CAD build for the part. Positions are in the model's coordinates, mm. A direction names the side the tool comes from. Coordinates: 2 decimals unless noted, no trailing zeros. Loops run counter-clockwise (first coordinate to the right, second up) from the corner with the lowest first, then second, coordinate; pieces in that order, holes last. Notation, with made-up numbers: (-38, 52) -> (-8, 52) arc R15 ccw to (-8, 65) -> close; hole circle Ø5 at (-38, 56.25). An arc over 180 degrees is marked (long way). Write item = value, one per line. Start each with the question number.
(1) Band-saw the part on C-C (y = 0). Write the cut outline in (x, z), and give its area (3 significant figures).
(2) Tool access for faces 5 (the face through (0, 21.5, 27)), 6 (the face through (5.109, 22.514, 37.026)): list every direction of +Z, -Z, +X, -X, +Y, -Y with a clear straight run to the whole face (end or side of a thin tool).
(3) Pull direction Z, two halves, no side cores. Call faces 1 (the face through (0, -21.5, 27)), 2 (the face through (-14.246, 22.514, 45.613)), 3 (the face through (0, 0, 0)), 4 (the face through (-10, 23, 49)): +Z half, -Z half, draft (parallel to the pull), parting line (faces both ways), or undercut.
(4) Band-saw the part on D-D (x = 14.25). Write the cut outline in (y, z).
(5) Drill centre lines: line 1 (Y direction, x = 3.5, z = 27); line 2 (Z direction, x = -13, y = 22); line 3 (Y direction, x = 14.25, z = 0.95). Where is each one in solid material? Low to high. Write a range as from..to.
(6) Band-saw the part on A-A (z = 18). Write the cut outline in (x, y).
(7) Flat gauge pins, fed straight in: P1, Ø7, axis at x = -13, z = 40, coming from the +Y side; P2, Ø2, axis at x = -16, y = 8, coming from the +Z side. Where does each tip first touch, or does it go through?
(8) Band-saw the part on B-B (x = -13). Write the cut outline in (y, z), and give its area (3 significant figures).
```python
from build123d import *

# Parameters (mm, degrees)
SKETCH1_W           = 48
SKETCH1_H           = 47
BOSS_EXTRUDE1_DEPTH = 49
SKETCH3_W           = 50
SKETCH3_H           = 43
CUT_EXTRUDE1_DEPTH  = 49
SKETCH4_R           = 9.25
CUT_EXTRUDE2_DEPTH  = 2
SKETCH5_R           = 5.75
SKETCH5_R_2         = 3
CUT_EXTRUDE3_DEPTH  = 2
SKETCH7_R           = 3
CUT_EXTRUDE4_DEPTH  = 2
FILLET1_R           = 25
FILLET2_R           = 6
FILLET3_R           = 3


with BuildPart() as part:
    # Sketch1 → Boss-Extrude1 (new body)
    with BuildSketch(Plane.XY):
        Rectangle(SKETCH1_W, SKETCH1_H)
    extrude(amount=BOSS_EXTRUDE1_DEPTH)

    # Sketch3 → Cut-Extrude1 (cut)
    with BuildSketch(Plane(origin=(24, 0, 0), x_dir=(0, 0, -1), z_dir=(1, 0, 0))):
        with Locations((-27, 0)):
            Rectangle(SKETCH3_W, SKETCH3_H)
    extrude(amount=-CUT_EXTRUDE1_DEPTH, mode=Mode.SUBTRACT)

    # Sketch4 → Cut-Extrude2 (cut)
    with BuildSketch(Plane.XY.offset(2)):
        with Locations((14.25, 0)):
            Circle(SKETCH4_R)
    extrude(amount=-CUT_EXTRUDE2_DEPTH, mode=Mode.SUBTRACT)

    # Sketch5 → Cut-Extrude3 (cut)
    with BuildSketch(Plane(origin=(0, 23.5, 0), x_dir=(1, 0, 0), z_dir=(0, 1, 0))):
        with Locations((-13, -40)):
            Circle(SKETCH5_R)
        with Locations((5.5, -40)):
            Circle(SKETCH5_R_2)
    extrude(amount=-CUT_EXTRUDE3_DEPTH, mode=Mode.SUBTRACT)

    # Sketch7 → Cut-Extrude4 (cut)
    with BuildSketch(Plane(origin=(0, -21.5, 0), x_dir=(1, 0, 0), z_dir=(0, 1, 0))):
        with Locations((5.5, -40)):
            Circle(SKETCH7_R)
        with Locations((-13, -40)):
            Circle(SKETCH7_R)
    extrude(amount=-CUT_EXTRUDE4_DEPTH, mode=Mode.SUBTRACT)

    # Fillet1
    fillet1_edges = [part.edges().sort_by_distance(p)[0] for p in [
        (24, 22.5, 49),
        (24, -22.5, 49),
    ]]
    fillet(fillet1_edges, radius=FILLET1_R)

    # Fillet2
    fillet2_edges = [part.edges().sort_by_distance(p)[0] for p in [
        (-24, 22.5, 49),
        (-24, -22.5, 49),
    ]]
    fillet(fillet2_edges, radius=FILLET2_R)

    # Fillet3
    fillet3_edges = [part.edges().sort_by_distance(p)[0] for p in [
        (0, 21.5, 2),
        (0, -21.5, 2),
    ]]
    fillet(fillet3_edges, radius=FILLET3_R)


solid = part.part
```
Findings below:
q1.outline = (-24, 0) -> (5, 0) -> (5, 2) -> (-24, 2) -> close; (23.5, 0) -> (24, 0) -> (24, 2) -> (23.5, 2) -> close
q1.area = 59.0 mm²
q2.face_5 = +Z, +X, -X
q2.face_6 = +Y, -Y
q3.face_1 = draft
q3.face_2 = undercut
q3.face_3 = -Z half
q3.face_4 = +Z half
q4.outline = (-23.5, 0) -> (-9.25, 0) -> (-9.25, 2) -> (-18.5, 2) arc R3 cw to (-21.5, 5) -> (-21.5, 43.81) -> (-23.5, 43.81) -> close; (9.25, 0) -> (23.5, 0) -> (23.5, 43.81) -> (21.5, 43.81) -> (21.5, 5) arc R3 cw to (18.5, 2) -> (9.25, 2) -> close
q5.line_1 = -23.5..-21.5, 21.5..23.5
q5.line_2 = 0..34.25, 45.75..49
q5.line_3 = -23.5..-9.25, 9.25..23.5
q6.outline = (-24, -23.5) -> (24, -23.5) -> (24, -21.5) -> (-24, -21.5) -> close; (-24, 21.5) -> (24, 21.5) -> (24, 23.5) -> (-24, 23.5) -> close
q7.P1 = -21.5
q7.P2 = 2
q8.outline = (-23.5, 0) -> (23.5, 0) -> (23.5, 34.25) -> (21.5, 34.25) -> (21.5, 5) arc R3 cw to (18.5, 2) -> (-18.5, 2) arc R3 cw to (-21.5, 5) -> (-21.5, 37) -> (-23.5, 37) -> close; (-23.5, 43) -> (-21.5, 43) -> (-21.5, 49) -> (-23.5, 49) -> close; (21.5, 45.75) -> (23.5, 45.75) -> (23.5, 49) -> (21.5, 49) -> close
q8.area = 251 mm²
